from build123d import *

# Parameters (mm, degrees)
F0_W     = 63.5
F0_H     = 457.2
F1_DEPTH = 50.8
F2_W     = 50.8
F2_H     = 19.05
F3_DEPTH = 457.2
F4_W     = 457.2
F4_H     = 6.35
F5_DEPTH = 6.35
F6_W     = 457.2
F6_H     = 3.175
F6_H_2   = 6.35
F7_DEPTH = 6.35
F8_W     = 457.2
F8_H     = 6.35
F9_DEPTH = 6.35


with BuildPart() as f1:
    # F0 (on Top) → F1 (new body)
    with BuildSketch(Plane.XY):
        with Locations((13.7360737771, 190.3568813264)):
            Rectangle(F0_W, F0_H)
    extrude(amount=F1_DEPTH)

    # F2 (on face) → F3 (cut)
    with BuildSketch(Plane.XZ.offset(38.2431186736)):
        with Locations((13.7360737771, 41.275)):
            Rectangle(F2_W, F2_H)
    extrude(amount=-F3_DEPTH, mode=Mode.SUBTRACT)

    # F4 (on face) → F5 (join)
    with BuildSketch(Plane.YZ.offset(-11.6639262229)):
        with Locations((190.3568813264, 41.787626493)):
            Rectangle(F4_W, F4_H)
    extrude(amount=F5_DEPTH)

    # F6 (on face) → F7 (join)
    with BuildSketch(Plane.YZ.offset(-5.3139262229)):
        with Locations((190.3568813264, 46.550126493)):
            Rectangle(F6_W, F6_H)
        with Locations((190.3568813264, 41.787626493)):
            Rectangle(F6_W, F6_H_2)
        with Locations((190.3568813264, 37.025126493)):
            Rectangle(F6_W, F6_H)
    extrude(amount=F7_DEPTH)

    # F8 (on face) → F9 (join)
    with BuildSketch(Plane(origin=(39.1360737771, 0, 0), x_dir=(0, -1, 0), z_dir=(-1, 0, 0))):
        with Locations((-190.3568813264, 41.275)):
            Rectangle(F8_W, F8_H)
    extrude(amount=F9_DEPTH)


solid = f1.part
The listing builds one solid part. Answer for the finished solid, in the listing's coordinates (mm). A direction names the side the tool comes from. Give positions to 0.01 mm unless a question says otherwise; leave off trailing zeros. Loops run counter-clockwise (first coordinate to the right, second up) from the corner with the lowest first, then second, coordinate; pieces in that order, holes last.
Item 1: A cutting plane is placed at B-B (x = 16.5). Give the vertices of the cut face in (y, z), then the cut area to 3 significant figures.
Derived:
outline: (-38.24, 0) - (418.96, 0) - (418.96, 31.75) - (-38.24, 31.75) - close
area: 14,500 mm2
Item 2: A tool of negligible diameter and unlimited length cuts with its end or side. For faces 4 (the flat face through (13, 187, 31.75)), 5 (the flat face through (13, 418.957, 19)), from which of +Z, -Z, +X, -X, +Y, -Y can it reach the whole face along a straight path? Write none if from no direction.
Derived:
face 4: +Y, -Y
face 5: +Z, -Z, +X, -X, +Y
Item 3: Find the intervals of material crossed by line 1 along X through (y, z) = (217, 48); line 2 along X through (y, z) = (-17, 39.5); line 3 along Z through (x, y) = (36.5, 368), in increasing order.
Derived:
line 1: x = -18.01 to -11.66, -5.31 to 1.04, 39.14 to 45.49
line 2: x = -18.01 to 1.04, 32.79 to 45.49
line 3: z = 0 to 31.75, 38.1 to 44.45
Item 4: Each of these flat-tipped pins is pushed along its axis until it touches: pin 1 Ø7 at (x, y) = (-3, 210.5) entering from +Z; pin 2 Ø8 at (x, y) = (13, 98.5) entering from +Z; pin 3 Ø1.9 at (x, y) = (-9.5, 164.5) entering from +Z. Where does it stop, or does it pass through?
Derived:
pin 1: stops at z = 48.14
pin 2: stops at z = 31.75
pin 3: stops at z = 44.96
Item 5: A cutting plane is placed at A-A (y = 43). Give the vertices of the cut face in (x, z).
Derived:
outline: (-18.01, 0) - (45.49, 0) - (45.49, 50.8) - (39.14, 50.8) - (39.14, 44.45) - (32.79, 44.45) - (32.79, 38.1) - (39.14, 38.1) - (39.14, 31.75) - (-11.66, 31.75) - (-11.66, 38.61) - (-5.31, 38.61) - (-5.31, 35.44) - (1.04, 35.44) - (1.04, 48.14) - (-5.31, 48.14) - (-5.31, 44.96) - (-11.66, 44.96) - (-11.66, 50.8) - (-18.01, 50.8) - close
Item 6: Determine the mould class of faces 1 (the flat face through (45.486, 187, 25)), 2 (the flat face through (13, 194, 0)), 3 (the flat face through (1.036, 187, 42)) for opening direction X: +X half, -X half, draft (parallel to the pull), parting line (faces both ways), or undercut.
Derived:
face 1: +X half
face 2: draft
face 3: undercut
